Could you check a few things on this model? Use its own coordinates, in mm. A direction names the side the tool comes from. Round coordinates to 2 decimals unless told otherwise and drop trailing zeros. Loops run counter-clockwise (first coordinate to the right, second up) from the corner with the lowest first, then second, coordinate; pieces in that order, holes last. Notation, with made-up numbers: (-19, -8) -> (14, -8) arc R29 ccw to (14, 27) -> close; hole circle Ø2 at (15.5, 61). An arc over 180 degrees is marked (long way). One line per item, written item: value.
```python
from build123d import *

# Parameters (mm, degrees)
MAINBLOCK_DEPTH               = 2.54
BOSS_EXTRUDE1_DEPTH           = 12.7
SKETCH3_R                     = 1.651
MOUNT_HOLES_DEPTH             = 124.889069578
FILLET1_R                     = 1.27
CHAMFER1_SIZE                 = 1.27
SKETCH4_W                     = 30.48
SKETCH4_H                     = 2.54
STABILIZER_MOUNT_CUTOUT_DEPTH = 5.08
FILLET2_R                     = 1.905


with BuildPart() as part:
    # Sketch1 → MainBlock (new body)
    with BuildSketch(Plane(origin=(0, 0, 0), x_dir=(1, 0, 0), z_dir=(0, 1, 0))):
        with BuildLine():
            Line((-99.441, 19.304), (99.441, 19.304))
            ThreePointArc((99.441, 19.304), (118.745, 0), (99.441, -19.304))
            Line((99.441, -19.304), (-99.441, -19.304))
            ThreePointArc((-99.441, -19.304), (-118.745, 0), (-99.441, 19.304))
        make_face()
    extrude(amount=MAINBLOCK_DEPTH)

    # Sketch2 → Boss-Extrude1 (add)
    with BuildSketch(Plane.XZ):
        with BuildLine():
            Line((-99.441, 21.844), (99.441, 21.844))
            ThreePointArc((99.441, 21.844), (121.285, 0), (99.441, -21.844))
            Line((99.441, -21.844), (-99.441, -21.844))
            ThreePointArc((-99.441, -21.844), (-121.285, 0), (-99.441, 21.844))
        make_face()
        with BuildLine():
            Line((99.441, 19.304), (-99.441, 19.304))
            ThreePointArc((-99.441, 19.304), (-118.745, 0), (-99.441, -19.304))
            Line((-99.441, -19.304), (99.441, -19.304))
            ThreePointArc((99.441, -19.304), (118.745, 0), (99.441, 19.304))
        make_face(mode=Mode.SUBTRACT)
    extrude(amount=-BOSS_EXTRUDE1_DEPTH)

    # Sketch3 → Mount-Holes (cut, through all)
    with BuildSketch(Plane.XZ):
        with Locations(Location((-84.201, 10.16, 0), (0, 0, 270))):
            Circle(SKETCH3_R)
        with Locations(Location((84.201, 10.16, 0), (0, 0, 90))):
            Circle(SKETCH3_R)
        with Locations(Location((84.201, -10.16, 0), (0, 0, 270))):
            Circle(SKETCH3_R)
        with Locations(Location((-84.201, -10.16, 0), (0, 0, 90))):
            Circle(SKETCH3_R)
    extrude(amount=-MOUNT_HOLES_DEPTH, mode=Mode.SUBTRACT)

    # Fillet1
    fillet1_edges = [part.edges().sort_by_distance(p)[0] for p in [
        (118.745, 2.54, 0),
        (0, 2.54, -19.304),
        (-118.745, 2.54, 0),
        (0, 2.54, 19.304),
    ]]
    fillet(fillet1_edges, radius=FILLET1_R)

    # Chamfer1
    chamfer1_edges = [part.edges().sort_by_distance(p)[0] for p in [
        (-121.285, 0, 0),
        (0, 0, -21.844),
        (121.285, 0, 0),
        (0, 0, 21.844),
    ]]
    chamfer(chamfer1_edges, length=CHAMFER1_SIZE)

    # Sketch4 → Stabilizer-Mount-Cutout (cut)
    with BuildSketch(Plane(origin=(0, 12.7, 0), x_dir=(1, 0, 0), z_dir=(0, 1, 0))):
        with Locations((-15.621, 20.574)):
            Rectangle(SKETCH4_W, SKETCH4_H)
    stabilizer_mount_cutout = extrude(amount=-STABILIZER_MOUNT_CUTOUT_DEPTH, mode=Mode.SUBTRACT)

    # Mirror1: Stabilizer-Mount-Cutout across plane
    add(stabilizer_mount_cutout.mirror(Plane.XY), mode=Mode.SUBTRACT)

    # Fillet2
    fillet2_edges = [part.edges().sort_by_distance(p)[0] for p in [
        (-30.861, 7.62, 20.574),
        (-0.381, 7.62, 20.574),
        (-0.381, 7.62, -20.574),
        (-30.861, 7.62, -20.574),
    ]]
    fillet(fillet2_edges, radius=FILLET2_R)


solid = part.part
```
Item 1: Will these pins go through, and if not, where does the flat tip stop? pin 1 Ø3 at (y, z) = (11, 20) entering from +X; pin 2 Ø4 at (x, z) = (84.201, 10.16) entering from +Y; pin 3 Ø3 at (y, z) = (10.5, 20) entering from -X; pin 4 Ø2.5 at (x, z) = (-84.201, -10.16) entering from +Y.
Output:
pin 1: stops at x = 111.06
pin 2: stops at y = 2.54
pin 3: stops at x = -111.06
pin 4: passes through
Item 2: For faces 4 (the face through (1, 8, 19.304)), 5 (the face through (-120.21, 0.2, -0.46)), which set-ups out of +Z, -Z, +X, -X, +Y, -Y let a thin tool reach every point of the face, with its end or its side?
Output:
face 4: +Y
face 5: -X, -Y
Item 3: If we mould it in two halves opening along Z, with no side actions, what happens to faces 1 (the face through (118.74, 8.19, -0.42)), 2 (the face through (120.21, 0.2, 0.46)), 3 (the face through (-1, 7, 21.844))? For each: released by +Z, released by -Z, zero draft, split by the parting line, or undercut.
Output:
face 1: undercut
face 2: split by the parting line
face 3: released by +Z
Item 4: If we section it at B-B on x = 64: List the corners of the cut face in (y, z) for me, plus the area to 3 significant figures.
Output:
outline: (0, -20.57) -> (1.27, -21.84) -> (12.7, -21.84) -> (12.7, -19.3) -> (3.81, -19.3) arc R1.27 cw to (2.54, -18.03) -> (2.54, 18.03) arc R1.27 cw to (3.81, 19.3) -> (12.7, 19.3) -> (12.7, 21.84) -> (1.27, 21.84) -> (0, 20.57) -> close
area: 162 mm²
Item 5: I need wall thicknesses on line 1 (X direction, y = 1.75, z = 10.16); line 2 (X direction, y = 1.5, z = -9.5); line 3 (Z direction, x = -32.5, y = 4). Which ranges of each line are inside material? Lowest first, please. Write a range as from..to.
Output:
line 1: x = -118.78..-85.85, -82.55..82.55, 85.85..118.78
line 2: x = -119.11..-85.71, -82.69..82.69, 85.71..119.11
line 3: z = -21.84..-19.3, 19.3..21.84
Item 6: If we section it at A-A on z = 0: List the corners of the cut face in (x, y) for me (3 decimals), plus the area to 3 significant figures.
Output:
outline: (-121.285, 1.27) -> (-120.015, 0) -> (120.015, 0) -> (121.285, 1.27) -> (121.285, 12.7) -> (118.745, 12.7) -> (118.745, 3.81) arc R1.27 cw to (117.475, 2.54) -> (-117.475, 2.54) arc R1.27 cw to (-118.745, 3.81) -> (-118.745, 12.7) -> (-121.285, 12.7) -> close
area: 667 mm²
